```python
from build123d import *

# Parameters (mm, degrees)
F0_W     = 38.3
F0_H     = 50.3
F0_W_2   = 28.3
F0_H_2   = 40.3
F2_DEPTH = 4
F3_DEPTH = 3
F4_R     = 5
F5_SIZE  = 2


with BuildPart() as f2:
    # F0 (on Top) → F2 (new body)
    with BuildSketch(Plane.XY):
        Rectangle(F0_W, F0_H)
        Rectangle(F0_W_2, F0_H_2, mode=Mode.SUBTRACT)
    extrude(amount=-F2_DEPTH)

    # F0 (on Top) → F3 (join)
    with BuildSketch(Plane.XY):
        Rectangle(F0_W, F0_H)
        Rectangle(F0_W_2, F0_H_2, mode=Mode.SUBTRACT)
        Rectangle(F0_W_2, F0_H_2)
    extrude(amount=F3_DEPTH)

    # F4
    f4_edges = [f2.edges().sort_by_distance(p)[0] for p in [
        (-19.15, -25.15, -0.5),
        (-19.15, 25.15, -0.5),
        (19.15, 25.15, -0.5),
        (19.15, -25.15, -0.5),
    ]]
    fillet(f4_edges, radius=F4_R)

    # F5
    f5_edges = [f2.edges().sort_by_distance(p)[0] for p in [
        (19.15, 0, 3),
        (17.685534, -23.685534, 3),
        (17.685534, 23.685534, 3),
        (0, -25.15, 3),
        (0, 25.15, 3),
        (-17.685534, -23.685534, 3),
        (-17.685534, 23.685534, 3),
        (-19.15, 0, 3),
    ]]
    chamfer(f5_edges, length=F5_SIZE)


solid = f2.part
```
Could you check a few things on this model? Use its own coordinates, in mm. A direction names the side the tool comes from. Coordinates: 2 decimals unless noted, no trailing zeros. Loops run counter-clockwise (first coordinate to the right, second up) from the corner with the lowest first, then second, coordinate; pieces in that order, holes last.
1) Thinking about a two-plate mould opening in X: for faces 3 (the face through (14.15, 0, -2)), 4 (the face through (0, -25.15, -2)), 5 (the face through (-18.16, 0.28, 1.99)), which applies, released by +X, released by -X, zero draft, split by the parting line, or undercut?
Reported:
face 3: undercut
face 4: zero draft
face 5: released by -X
2) Imagine slicing it at D-D (y = -13). List the corners of the cut face in (x, z) for me, and give its area (3 significant figures).
Reported:
outline: (-19.15, -4) - (-14.15, -4) - (-14.15, 0) - (14.15, 0) - (14.15, -4) - (19.15, -4) - (19.15, 1) - (17.15, 3) - (-17.15, 3) - (-19.15, 1) - close
area: 151 mm2
3) Imagine slicing it at A-A (z = 2). List the corners of the cut face in (x, y) for me, and give its area (3 significant figures).
Reported:
outline: (-18.15, -20.15) arc R4 ccw to (-14.15, -24.15) - (14.15, -24.15) arc R4 ccw to (18.15, -20.15) - (18.15, 20.15) arc R4 ccw to (14.15, 24.15) - (-14.15, 24.15) arc R4 ccw to (-18.15, 20.15) - close
area: 1,740 mm2
4) Please list where these lines run through material, in increasing order: line 1 along Y through (x, z) = (-1, -0.25); line 2 along X through (y, z) = (4, -3.25); line 3 along Z through (x, y) = (-11.5, -6).
Reported:
line 1: y = -25.15 to -20.15, 20.15 to 25.15
line 2: x = -19.15 to -14.15, 14.15 to 19.15
line 3: z = 0 to 3
5) Will this pin go through, and if not, where does the flat tip stop? pin 1 Ø14 at (x, y) = (4, 6.5) entering from -Z.
Reported:
pin 1: stops at z = 0
6) Which directions (+Z, -Z, +X, -X, +Y, -Y) give clear straight access to the entire face, cutting with the end or side of a thin tool? Please do faces 1 (the face through (-14.15, 0, -2)), 2 (the face through (17.65, -23.72, -1.46)).
Reported:
face 1: -Z
face 2: +Z, -Z, +X, -Y
7) Imagine slicing it at B-B (z = -0.75). List the corners of the cut face in (x, y) for me, and give its area (3 significant figures).
Reported:
outline: (-19.15, -20.15) arc R5 ccw to (-14.15, -25.15) - (14.15, -25.15) arc R5 ccw to (19.15, -20.15) - (19.15, 20.15) arc R5 ccw to (14.15, 25.15) - (-14.15, 25.15) arc R5 ccw to (-19.15, 20.15) - close; hole (-14.15, -20.15) - (14.15, -20.15) - (14.15, 20.15) - (-14.15, 20.15) - close
area: 765 mm2
8) Imagine slicing it at C-C (x = -4). List the corners of the cut face in (y, z) for me.
Reported:
outline: (-25.15, -4) - (-20.15, -4) - (-20.15, 0) - (20.15, 0) - (20.15, -4) - (25.15, -4) - (25.15, 1) - (23.15, 3) - (-23.15, 3) - (-25.15, 1) - close
